Here's the drawing with two shaded views (mm, measured from the low corner). I have some questions. Coordinates: 2 decimals unless noted, no trailing zeros. Write each loop counter-clockwise with the first axis right and the second up, starting at its lowest first coordinate (ties: lowest second). Pieces come first, ordered by that corner, then holes. Notation, with made-up numbers: M -34,-26 L -7,-26 A14 ccw -7,-18 Z; hole C 88,-30.5 d9. An arc over 180 degrees is marked long. Use one line per item in the form item = value. Start each with the question number.
1. I'm going to push a flat-ended pin straight in: pin 1 Ø3 at (x, y) = (4.5, 4) entering from +Z. Where does the tip first touch, or does it pass through?
2. I want a section at C-C, the plane z = 8. List the corners of the cut face in (x, y) for me.
3. I want a section at A-A, the plane y = 3. List the corners of the cut face in (x, z) for me.
4. Please list where these lines run through material, in increasing order: line 1 along X through (y, z) = (3, 6.75); line 2 along Z through (x, y) = (5.2, 4.4); line 3 along X through (y, z) = (2.05, 1.25). Write a range as [from, to].
5. Thinking about a two-plate mould opening in X: for the marked faces 1, 2 and 3, which applies, released by +X, released by -X, zero draft, split by the parting line, or undercut?
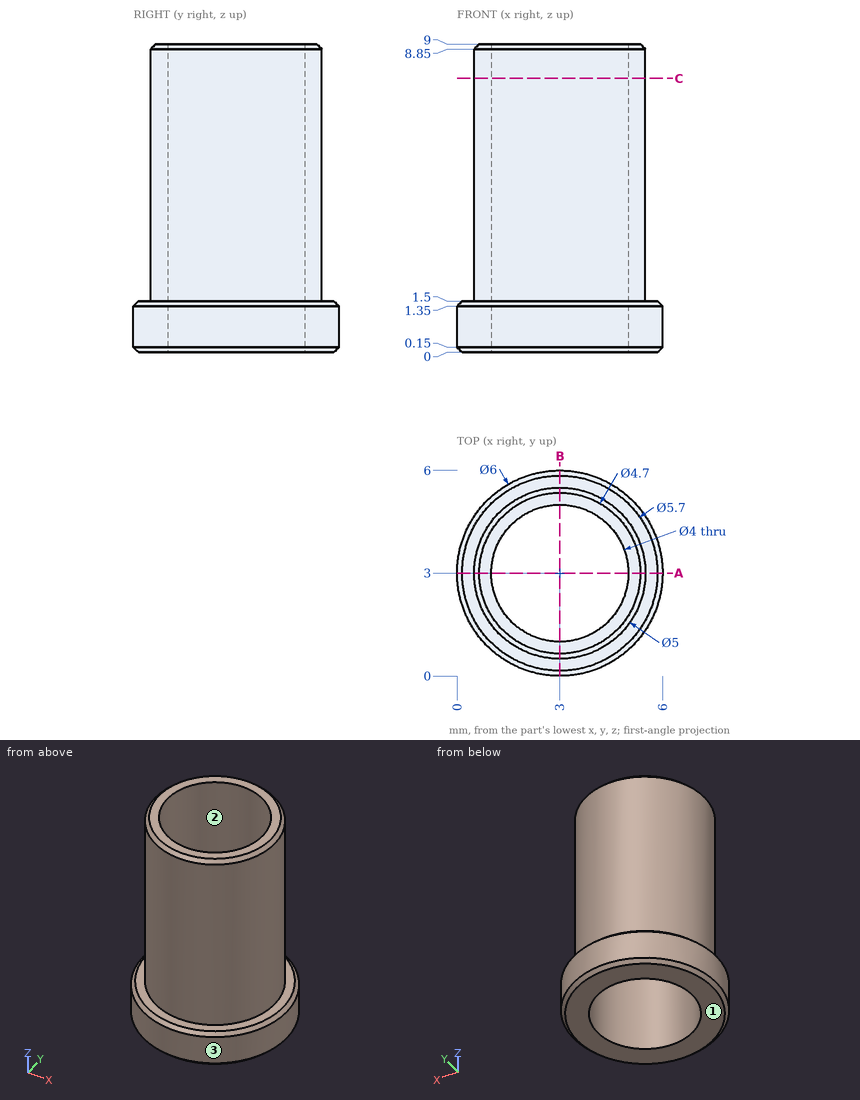
Answer list:
q1.pin_1 = 9
q2.outline = C 3,3 d5; hole C 3,3 d4
q3.outline = M 0,0.15 L 0.15,0 L 1,0 L 1,9 L 0.65,9 L 0.5,8.85 L 0.5,1.5 L 0.15,1.5 L 0,1.35 Z; M 5,0 L 5.85,0 L 6,0.15 L 6,1.35 L 5.85,1.5 L 5.5,1.5 L 5.5,8.85 L 5.35,9 L 5,9 Z
q4.line_1 = [0.5, 1], [5, 5.5]
q4.line_2 = [0, 1.5]
q4.line_3 = [0.15, 1.24], [4.76, 5.85]
q5.face_1 = zero draft
q5.face_2 = undercut
q5.face_3 = split by the parting line
